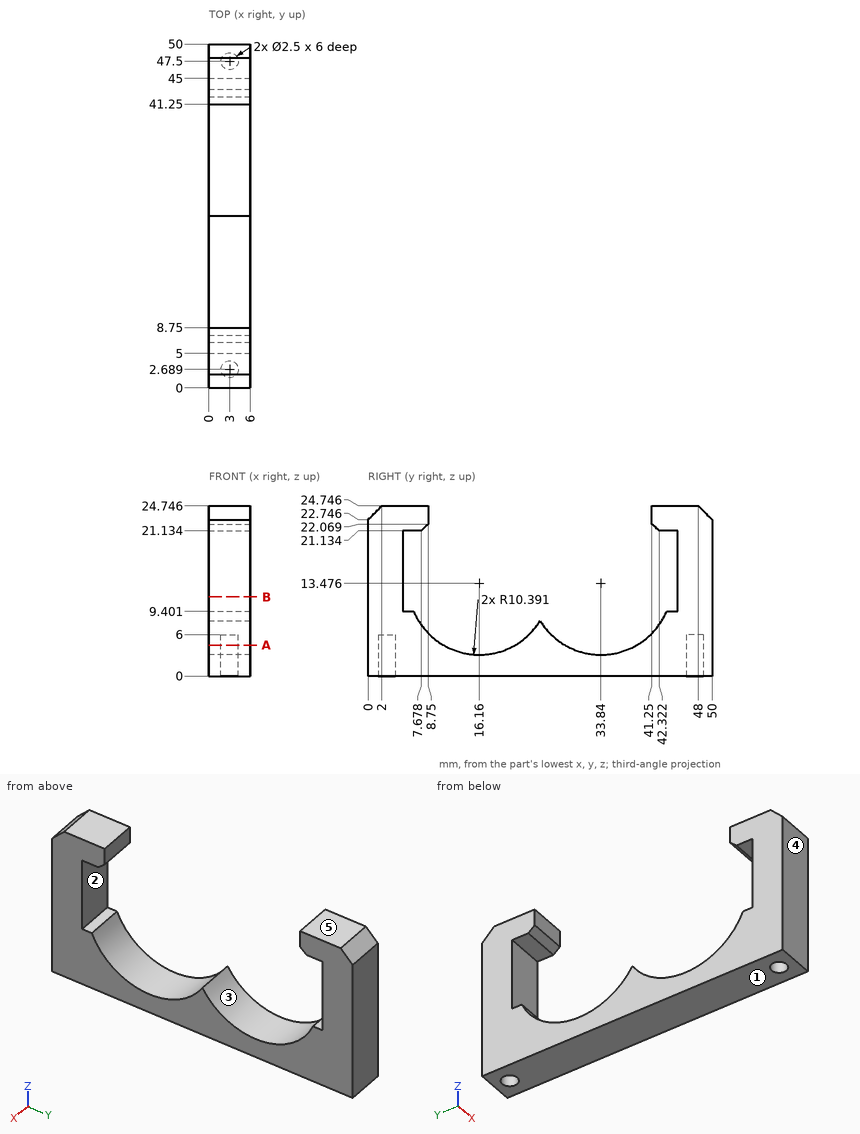
Verification items for this drawing (mm, ordinates from the low corner). A direction names the side the tool comes from. Give positions to 0.01 mm unless a question says otherwise; leave off trailing zeros. Loops run counter-clockwise (first coordinate to the right, second up) from the corner with the lowest first, then second, coordinate; pieces in that order, holes last.
1. Go/stop test with flat-tipped pins: P1, Ø8, axis at y = 10.5, z = 14.5, coming from the -X side; P2, Ø1.2, axis at x = 3, y = 2.5, coming from the -Z side; P3, Ø1, axis at x = 3.5, y = 22.5, coming from the +Z side (1 decimal); P4, Ø0.8, axis at x = 3, z = 23.5, coming from the -Y side (1 decimal). Record where each tip stops, or that it passes through.
Derived:
P1: passes through
P2: stops at z = 6
P3: stops at z = 5.7
P4: stops at y = 0.4
2. Material ranges on probe 1 along Y at (x, z) = (1.6, 13.5); probe 2 along Z at (x, y) = (1.5, 44) (1 decimal); probe 3 along Y at (x, z) = (2.15, 7.75), recorded low to high.
Derived:
probe 1: y = 0 to 5, 45 to 50
probe 2: z = 0 to 9.4, 21.1 to 24.7
probe 3: y = 0 to 7.49, 24.83 to 25.17, 42.51 to 50
3. Cross-section at B-B on z = 11.5. Record the cut outline in (x, y).
Derived:
outline: (0, 0) - (6, 0) - (6, 5) - (0, 5) - close; (0, 45) - (6, 45) - (6, 50) - (0, 50) - close
4. Tool access check on the marked faces 1 and 2. Record the directions out of +Z, -Z, +X, -X, +Y, -Y that give a thin tool (end or side, any length) a straight path to the whole face; none if there is none.
Derived:
face 1: -Z, +X, -X, +Y, -Y
face 2: +X, -X
5. Release check for a two-part mould opening along Y. For the marked faces 3, 4 and 5 record: +Y half, -Y half, draft (parallel to the pull), parting line (faces both ways), or undercut.
Derived:
face 3: undercut
face 4: -Y half
face 5: draft
6. Cross-section at A-A on z = 4.5. Count the separate pieces of the cut face and the enclosed holes in it.
Derived:
separate pieces: 3
enclosed holes: 2
